Model file for the job. Use its own axes, mm. A direction names the side the tool comes from. Round coordinates to 2 decimals unless told otherwise and drop trailing zeros. Order: outer loops, then holes, each group sorted by start corner. A loop starts at its lowest first (then second) coordinate and runs counter-clockwise, first axis right, second up. Notation, with made-up numbers: (32.25, 12) -> (61.25, 12) arc R24 ccw to (61.25, 23) -> close; hole circle Ø9 at (-19, -1). An arc over 180 degrees is marked (long way). Answer as CSV lines item,"result".
```python
from build123d import *

# Parameters (mm, degrees)
BOSS_EXTRUDE1_DEPTH     = 6
FILLET1_R               = 5
FILLET2_R               = 20
SKETCH2_W               = 6
SKETCH2_H               = 10
CUT_EXTRUDE1_DEPTH      = 1
CUT_EXTRUDE1_DEPTH_BACK = 7


with BuildPart() as part:
    # Sketch1 → Boss-Extrude1 (new body)
    with BuildSketch(Plane.XY):
        Polygon((70, 0), (-70, 0), (-97.66666667, -8), (-147.66666667, -8), (-147.66666667, -20), (-122.66666667, -20), (-122.66666667, -26), (-112.66666667, -26), (-112.66666667, -20), (112.66666667, -20), (112.66666667, -26), (122.66666667, -26), (122.66666667, -20), (147.66666667, -20), (147.66666667, -8), (97.66666667, -8), align=None)
    extrude(amount=BOSS_EXTRUDE1_DEPTH)

    # Fillet1
    fillet1_edges = [part.edges().sort_by_distance(p)[0] for p in [
        (-147.66666667, -8, 3),
        (147.66666667, -8, 3),
    ]]
    fillet(fillet1_edges, radius=FILLET1_R)

    # Fillet2
    fillet2_edges = [part.edges().sort_by_distance(p)[0] for p in [
        (-97.66666667, -8, 3),
        (-70, 0, 3),
        (70, 0, 3),
        (97.66666667, -8, 3),
    ]]
    fillet(fillet2_edges, radius=FILLET2_R)

    # Sketch2 → Cut-Extrude1 (cut, two sides)
    with BuildSketch(Plane.XY.offset(6)) as cut_extrude1_sk:
        with Locations((0, -15)):
            Rectangle(SKETCH2_W, SKETCH2_H)
    extrude(amount=CUT_EXTRUDE1_DEPTH, mode=Mode.SUBTRACT)
    extrude(cut_extrude1_sk.sketch, amount=-CUT_EXTRUDE1_DEPTH_BACK, mode=Mode.SUBTRACT)


solid = part.part
```
Q1. Saw through at B-B (x = -105). Write the cut outline in (y, z).
Checks:
outline,"(-20, 0) -> (-8, 0) -> (-8, 6) -> (-20, 6) -> close"
Q2. Saw through at A-A (z = 5). Write the cut outline in (x, y), plus the area to 3 significant figures.
Checks:
outline,"(-147.67, -20) -> (-122.67, -20) -> (-122.67, -26) -> (-112.67, -26) -> (-112.67, -20) -> (-3, -20) -> (-3, -10) -> (3, -10) -> (3, -20) -> (112.67, -20) -> (112.67, -26) -> (122.67, -26) -> (122.67, -20) -> (147.67, -20) -> (147.67, -13) arc R5 ccw to (142.67, -8) -> (100.5, -8) arc R20 cw to (94.94, -7.21) -> (72.72, -0.79) arc R20 ccw to (67.17, 0) -> (-67.17, 0) arc R20 ccw to (-72.72, -0.79) -> (-94.94, -7.21) arc R20 cw to (-100.5, -8) -> (-142.67, -8) arc R5 ccw to (-147.67, -13) -> close"
area,"4,930 mm²"
Q3. Wall check: L1, parallel to X at y = -15.25, z = 5.05; L2, parallel to X at y = -21.5, z = 2.5; L3, parallel to Y at x = -51, z = 3.2. Give the ranges that are in metal, low to high. Write a range as [from, to].
Checks:
L1,"[-147.67, -3], [3, 147.67]"
L2,"[-122.67, -112.67], [112.67, 122.67]"
L3,"[-20, 0]"
Q4. Flat gauge pins, fed straight in: pin 1 (3 mm diameter, centred on x = -83, z = 3, fed in from +Y); pin 2 (3 mm diameter, centred on x = -113.5, z = 3, fed in from +Y); pin 3 (3 mm diameter, centred on y = -22.5, z = 2, fed in from +X). Where does each tip first touch, or does it go through?
Checks:
pin 1,"y = -3.33"
pin 2,"y = -8"
pin 3,"x = 122.67"
Q5. Tool access for faces 1 (the flat face through (-121, -8, 3)), 2 (the flat face through (-59, -20, 3)), 3 (the flat face through (135, -20, 3)), 4 (the flat face through (122, -8, 3)), 5 (the flat face through (-135, -20, 3)): list every direction of +Z, -Z, +X, -X, +Y, -Y with a clear straight run to the whole face (end or side of a thin tool).
Checks:
face 1,"+Z, -Z, -X, +Y"
face 2,"+Z, -Z, -Y"
face 3,"+Z, -Z, +X, -Y"
face 4,"+Z, -Z, +X, +Y"
face 5,"+Z, -Z, -X, -Y"
Q6. Saw through at C-C (x = -29). Write the cut outline in (y, z), plus the area to 3 significant figures.
Checks:
outline,"(-20, 0) -> (0, 0) -> (0, 6) -> (-20, 6) -> close"
area,"120 mm²"
